Autodesk Inventor part; units mm, degrees
ref_plane "YZ Plane" through (0, 0, 0) normal (1, 0, 0) x (0, 1, 0)
ref_plane "XZ Plane" through (0, 0, 0) normal (0, 1, 0) x (-1, 0, 0)
ref_plane "XY Plane" through (0, 0, 0) normal (0, 0, 1) x (1, 0, 0)
sketch "Skizze1" plane through (0, 0, 0) normal (0, 0, 1) x (1, 0, 0)
  line L0 (0, 0) -> (166, 0)
  line L1 (166, 0) -> (166, 80)
  line L2 (166, 80) -> (0, 80)
  line L3 (0, 80) -> (0, 0)
  dimension "d0" = 80
  dimension "d1" = 166
extrude "Extrusion1" add sketch "Skizze1" along normal blind 2
sketch "Skizze2" plane through (0, 0, 0) normal (0, 0, -1) x (-1, 0, 0)
  line L0 (-2.2, 77.8) -> (-12, 77.8)
  line L1 (-12, 77.8) -> (-12, 68)
  line L2 (-12, 68) -> (-2.2, 68)
  line L3 (-2.2, 68) -> (-2.2, 77.8)
  line L4 (0, 80) -> (0, 0)
  line L5 (-166, 80) -> (0, 80)
  line L6 (0, 80) -> (0, 0)
  line L7 (0, 40) -> (18.01, 40)
  line L8 (-166, 80) -> (0, 80)
  line L9 (-83, 80) -> (-83, 127.491)
  line L10 (-2.2, 2.2) -> (-12, 2.2)
  line L11 (-12, 2.2) -> (-12, 12)
  line L12 (-12, 12) -> (-2.2, 12)
  line L13 (-2.2, 12) -> (-2.2, 2.2)
  line L14 (-163.8, 77.8) -> (-154, 77.8)
  line L15 (-154, 77.8) -> (-154, 68)
  line L16 (-154, 68) -> (-163.8, 68)
  line L17 (-163.8, 68) -> (-163.8, 77.8)
  line L18 (-166, 80) -> (-166, 0)
  line L19 (-166, 80) -> (-166, 0)
  line L20 (-163.8, 2.2) -> (-154, 2.2)
  line L21 (-154, 2.2) -> (-154, 12)
  line L22 (-154, 12) -> (-163.8, 12)
  line L23 (-163.8, 12) -> (-163.8, 2.2)
  point P0 (-166, 40)
  dimension "d4" = 2.2
  dimension "d5" = 2.2
  dimension "d6" = 9.8
  dimension "d7" = 9.8
  dimension "d8" = 40
extrude "Extrusion2" add sketch "Skizze2" along normal blind 5
sketch "Skizze3" plane through (0, 0, 2) normal (0, 0, 1) x (1, 0, 0)
  line L0 (0, 80) -> (0, 0)
  line L1 (0, 0) -> (166, 0)
  line L2 (0, 80) -> (0, 0)
  line L3 (0, 40) -> (-51.158, 40)
  line L4 (0, 0) -> (166, 0)
  line L5 (83, 0) -> (83, -45.9243)
  line L6 (166, 80) -> (166, 0)
  line L7 (166, 0) -> (0, 0)
  line L8 (166, 80) -> (166, 0)
  line L9 (166, 40) -> (217.158, 40)
  line L10 (166, 0) -> (0, 0)
  point P0 (7, 7)
  point P1 (7, 73)
  point P2 (159, 7)
  point P3 (159, 73)
  dimension "d11" = 7
  dimension "d12" = 7
hole "Bohrung1" at (7, 7, 2) at (7, 73, 2) at (159, 73, 2) at (159, 7, 2) direction (0, 0, -1) diameter 3.5 depth 8 tip angle 118
sketch "Skizze4" plane through (0, 0, 2) normal (0, 0, 1) x (1, 0, 0)
  circle A0 centre (7, 7) radius 1.75
  circle A1 centre (7, 73) radius 1.75
  circle A2 centre (159, 7) radius 1.75
  circle A3 centre (159, 73) radius 1.75
  point P0 (0, 0)
hole "Bohrung2" at (7, 7, 2) at (7, 73, 2) at (159, 7, 2) at (159, 73, 2) direction (0, 0, -1) diameter 8 depth 5 tip angle 118
properties part number "TimDeckel"
Model file for the job. Use its own axes, mm. A direction names the side the tool comes from. Round coordinates to 2 decimals unless told otherwise and drop trailing zeros. Order: outer loops, then holes, each group sorted by start corner. A loop starts at its lowest first (then second) coordinate and runs counter-clockwise, first axis right, second up. Notation, with made-up numbers: M -0.75,-36.75 L 36.25,-36.75 A10 cw 36.25,-22.75 Z; hole C 26.25,30.25 d3. An arc over 180 degrees is marked long. Use CSV: the item, a comma, the result in double quotes.
Item 1: Saw through at B-B (x = 7). List the corners of the cut face in (y, z).
Worked answers:
outline,"M 0,0 L 2.2,0 L 2.2,-5 L 5.25,-5 L 5.25,-4.35 L 3,-3 L 3,2 L 0,2 Z; M 8.75,-5 L 12,-5 L 12,0 L 68,0 L 68,-5 L 71.25,-5 L 71.25,-4.35 L 69,-3 L 69,2 L 11,2 L 11,-3 L 8.75,-4.35 Z; M 74.75,-5 L 77.8,-5 L 77.8,0 L 80,0 L 80,2 L 77,2 L 77,-3 L 74.75,-4.35 Z"
Item 2: Saw through at C-C (y = 7). List the corners of the cut face in (x, z).
Worked answers:
outline,"M 0,0 L 2.2,0 L 2.2,-5 L 5.25,-5 L 5.25,-4.35 L 3,-3 L 3,2 L 0,2 Z; M 8.75,-5 L 12,-5 L 12,0 L 154,0 L 154,-5 L 157.25,-5 L 157.25,-4.35 L 155,-3 L 155,2 L 11,2 L 11,-3 L 8.75,-4.35 Z; M 160.75,-5 L 163.8,-5 L 163.8,0 L 166,0 L 166,2 L 163,2 L 163,-3 L 160.75,-4.35 Z"
Item 3: Probe probe 1 along Y at (x, z) = (7, -0.6); probe 2 along X at (y, z) = (7, -4.65); probe 3 along X at (y, z) = (73, -0.1). List the from-to ranges inside material, lowest first.
Worked answers:
probe 1,"2.2 to 3, 11 to 12, 68 to 69, 77 to 77.8"
probe 2,"2.2 to 5.25, 8.75 to 12, 154 to 157.25, 160.75 to 163.8"
probe 3,"2.2 to 3, 11 to 12, 154 to 155, 163 to 163.8"
Item 4: Saw through at D-D (y = 19.5). List the corners of the cut face in (x, z), plus the area to 3 significant figures.
Worked answers:
outline,"M 0,0 L 166,0 L 166,2 L 0,2 Z"
area,"332 mm²"
Item 5: Saw through at A-A (z = -1.75). List the corners of the cut face in (x, y).
Worked answers:
outline,"M 2.2,2.2 L 12,2.2 L 12,12 L 2.2,12 Z; M 2.2,68 L 12,68 L 12,77.8 L 2.2,77.8 Z; M 154,2.2 L 163.8,2.2 L 163.8,12 L 154,12 Z; M 154,68 L 163.8,68 L 163.8,77.8 L 154,77.8 Z; hole C 7,7 d8; hole C 7,73 d8; hole C 159,7 d8; hole C 159,73 d8"
Item 6: Which spindle directions (+Z, -Z, +X, -X, +Y, -Y) get a long thin tool onto all of the face, cutting with end or side? Do faces 4 (the face through (9.4, 10.2, -0.5)), 5 (the face through (154, 7, -2)), 6 (the face through (2.2, 7, -2)), 7 (the face through (7, 2.2, -2)). Say none if no direction does.
Worked answers:
face 4,"+Z"
face 5,"-Z, +Y, -Y"
face 6,"-Z, -X, +Y, -Y"
face 7,"-Z, +X, -X, -Y"
Item 7: Pin check, flat tips, straight feed: pin 1 (1.5 mm diameter, centred on y = 7.5, z = -1.5, fed in from -X); pin 2 (4 mm diameter, centred on y = 6.5, z = -2.5, fed in from +X); pin 3 (2.5 mm diameter, centred on x = 159, z = -3.5, fed in from -Y); pin 4 (3 mm diameter, centred on x = 7, y = 73, fed in from +Z). Stop position of each tip, or through.
Worked answers:
pin 1,"x = 2.2"
pin 2,"x = 163.8"
pin 3,"y = 2.2"
pin 4,"through"
Item 8: Pull direction X, two halves, no side cores. Call faces 1 (the face through (155.034, 73.521, -0.535)), 2 (the face through (2.2, 73, -2)), 3 (the face through (157, 7, -5)): released by +X, released by -X, zero draft, split by the parting line, or undercut.
Worked answers:
face 1,"undercut"
face 2,"released by -X"
face 3,"zero draft"
